```python
from build123d import *

# Parameters (mm, degrees)
F0_W     = 71.12
F0_H     = 71.12
F1_DEPTH = 25.4
F2_R     = 31.75
F3_DEPTH = 12.7
F4_R     = 19.05
F5_DEPTH = 12.7
F6_R     = 1.905
F7_DEPTH = 25.401
F9_DEPTH = 12.7
F10_R    = 5.08


with BuildPart() as f1:
    # F0 (on Top) → F1 (new body)
    with BuildSketch(Plane.XY):
        Rectangle(F0_W, F0_H)
    extrude(amount=F1_DEPTH)

    # F2 (on face) → F3 (cut)
    with BuildSketch(Plane.XY.offset(25.4)):
        Circle(F2_R)
    extrude(amount=-F3_DEPTH, mode=Mode.SUBTRACT)

    # F4 (on face) → F5 (join)
    with BuildSketch(Plane.XY.offset(12.7)):
        Circle(F4_R)
    extrude(amount=F5_DEPTH)

    # F6 (on face) → F7 (cut, through all)
    with BuildSketch(Plane.XY.offset(25.4)):
        with Locations((-26.9407683632, -26.9407683632)):
            Circle(F6_R)
        with Locations((-26.9407683632, 26.9407683632)):
            Circle(F6_R)
        with Locations((26.9407683632, 26.9407683632)):
            Circle(F6_R)
    extrude(amount=-F7_DEPTH, mode=Mode.SUBTRACT)

    # F8 (on face) → F9 (cut)
    with BuildSketch(Plane.XY.offset(25.4)):
        with BuildLine():
            ThreePointArc((18.5544223232, -4.3169332), (19.05, 0), (18.5544223232, 4.3169332))
            Line((18.5544223232, 4.3169332), (-18.5544223232, 4.3169332))
            ThreePointArc((-18.5544223232, 4.3169332), (-19.05, 0), (-18.5544223232, -4.3169332))
            Line((-18.5544223232, -4.3169332), (18.5544223232, -4.3169332))
        make_face()
    extrude(amount=-F9_DEPTH, mode=Mode.SUBTRACT)

    # F10
    f10_edges = [f1.edges().sort_by_distance(p)[0] for p in [
        (-35.56, -35.56, 12.7),
        (0, -35.56, 0),
        (-35.56, 0, 0),
        (0, 35.56, 0),
        (35.56, 0, 0),
        (35.56, -35.56, 12.7),
        (35.56, 35.56, 12.7),
        (-35.56, 35.56, 12.7),
    ]]
    fillet(f10_edges, radius=F10_R)


solid = f1.part
```
Model file for the job. Use its own axes, mm. A direction names the side the tool comes from. Coordinates: 2 decimals unless noted, no trailing zeros. Write each loop counter-clockwise with the first axis right and the second up, starting at its lowest first coordinate (ties: lowest second). Pieces come first, ordered by that corner, then holes. Notation, with made-up numbers: (18, 34.5) - (60, 34.5) arc R36 cw to (60, 69.5) - close; hole circle Ø10 at (66, 69). An arc over 180 degrees is marked (long way). Use a Markdown table: item, result. Add a question column.
Item 1: Band-saw the part on A-A, the plane z = 15.25. Write the cut outline in (x, y) (3 decimals), and give its area (3 significant figures).
Item 2: Band-saw the part on B-B, the plane y = 0. Write the cut outline in (x, z), and give its area (3 significant figures).
Item 3: 3-axis set-ups, long thin cutter, end or side, ignore diameter. For faces 1 (the face through (0, 4.317, 19)), 2 (the face through (34.032, 34.111, 15.382)): which of +Z, -Z, +X, -X, +Y, -Y reach the whole face in a straight line?
Item 4: Band-saw the part on D-D, the plane z = 4. Write the cut outline in (x, y) (3 decimals), and give its area (3 significant figures).
Item 5: Band-saw the part on C-C, the plane x = -20. Write the cut outline in (y, z), and give its area (3 significant figures).
Item 6: Two-plate mould, pull along Y, no slides. Class faces 3 (the face through (-34.111, -34.032, 15.382)), 4 (the face through (-34.111, 34.032, 15.382)), 5 (the face through (-0.358, -19.047, 18.961)): pulls with the +Y half, pulls with the -Y half, needs draft (parallel to the pull), parting line crosses it, or undercut.
Item 7: Drill centre lines: line 1 along Y through (x, z) = (-6, 13.75); line 2 along X through (y, z) = (-27, 23.75); line 3 along X through (y, z) = (9, 13.5). Where is each one in solid material? Low to high.
Item 8: Drop a flat-ended pin along its axis: pin 1 (1 mm diameter, centred on y = 27, z = 3.5, fed in from -X). Give the stop position or say it passes through.
A:
| question | item | result |
|---|---|---|
| 1 | outline | (-35.56, -30.48) arc R5.08 ccw to (-30.48, -35.56) - (30.48, -35.56) arc R5.08 ccw to (35.56, -30.48) - (35.56, 30.48) arc R5.08 ccw to (30.48, 35.56) - (-30.48, 35.56) arc R5.08 ccw to (-35.56, 30.48) - close; (-18.554, -4.317) arc R19.05 ccw to (18.554, -4.317) - close; (-18.554, 4.317) - (18.554, 4.317) arc R19.05 ccw to start; hole circle Ø63.5 at (0, 0); hole circle Ø3.81 at (-26.941, -26.941); hole circle Ø3.81 at (-26.941, 26.941); hole circle Ø3.81 at (26.941, 26.941) |
| 1 | area | 2,650 mm² |
| 2 | outline | (-35.56, 5.08) arc R5.08 ccw to (-30.48, 0) - (30.48, 0) arc R5.08 ccw to (35.56, 5.08) - (35.56, 25.4) - (31.75, 25.4) - (31.75, 12.7) - (-31.75, 12.7) - (-31.75, 25.4) - (-35.56, 25.4) - close |
| 2 | area | 989 mm² |
| 3 | face 1 | +Z |
| 3 | face 2 | +Z, -Z, +X, +Y |
| 4 | outline | (-35.444, -30.48) arc R4.964 ccw to (-30.48, -35.444) - (30.48, -35.444) arc R4.964 ccw to (35.444, -30.48) - (35.444, 30.48) arc R4.964 ccw to (30.48, 35.444) - (-30.48, 35.444) arc R4.964 ccw to (-35.444, 30.48) - close; hole circle Ø3.81 at (-26.941, -26.941); hole circle Ø3.81 at (-26.941, 26.941); hole circle Ø3.81 at (26.941, 26.941) |
| 4 | area | 4,970 mm² |
| 5 | outline | (-35.56, 5.08) arc R5.08 ccw to (-30.48, 0) - (30.48, 0) arc R5.08 ccw to (35.56, 5.08) - (35.56, 25.4) - (24.66, 25.4) - (24.66, 12.7) - (-24.66, 12.7) - (-24.66, 25.4) - (-35.56, 25.4) - close |
| 5 | area | 1,170 mm² |
| 6 | face 3 | pulls with the -Y half |
| 6 | face 4 | pulls with the +Y half |
| 6 | face 5 | undercut |
| 7 | line 1 | y = -35.56 to -31.18, -18.08 to -4.32, 4.32 to 18.08, 31.18 to 35.56 |
| 7 | line 2 | x = -35.56 to -28.84, -25.04 to -16.71, 16.71 to 35.56 |
| 7 | line 3 | x = -35.56 to -30.45, -16.79 to 16.79, 30.45 to 35.56 |
| 8 | pin 1 | stops at x = -35.44 |
